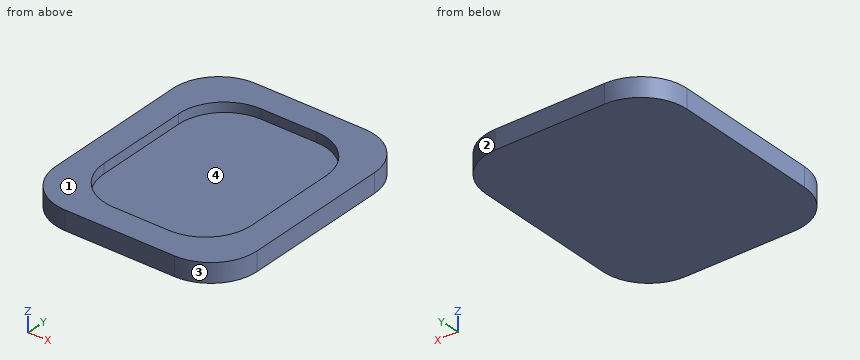
from build123d import *

# Parameters (mm, degrees)
F1_DEPTH = 5
F2_W     = 38.5
F2_H     = 48.5
F3_DEPTH = 2.5
F4_R     = 12


with BuildPart() as f1:
    # F0 (on Top) → F1 (new body)
    with BuildSketch(Plane.XY):
        with BuildLine():
            Line((40.5, 0), (12, 0))
            ThreePointArc((12, 0), (3.514719, -3.514719), (0, -12))
            Line((0, -12), (0, -50.5))
            ThreePointArc((0, -50.5), (3.514719, -58.985281), (12, -62.5))
            Line((12, -62.5), (40.5, -62.5))
            ThreePointArc((40.5, -62.5), (48.985281, -58.985281), (52.5, -50.5))
            Line((52.5, -50.5), (52.5, -12))
            ThreePointArc((52.5, -12), (48.985281, -3.514719), (40.5, 0))
        make_face()
    extrude(amount=F1_DEPTH)

    # F2 (on face) → F3 (cut)
    with BuildSketch(Plane.XY.offset(5)):
        with Locations((26.25, -31.25)):
            Rectangle(F2_W, F2_H)
    extrude(amount=-F3_DEPTH, mode=Mode.SUBTRACT)

    # F4
    f4_edges = [f1.edges().sort_by_distance(p)[0] for p in [
        (7, -7, 3.75),
        (45.5, -7, 3.75),
        (7, -55.5, 3.75),
        (45.5, -55.5, 3.75),
    ]]
    fillet(f4_edges, radius=F4_R)


solid = f1.part
Geometry check sheet. Reference: the model listing, model coordinates, mm. Face numbers are marked on the shaded views. Round coordinates to 2 decimals unless told otherwise and drop trailing zeros. Order: outer loops, then holes, each group sorted by start corner. A loop starts at its lowest first (then second) coordinate and runs counter-clockwise, first axis right, second up. Notation, with made-up numbers: M 23,19.25 L 65,19.25 A33 ccw 65,51.25 Z; hole C -14.5,16.25 d2. An arc over 180 degrees is marked long. Write each question's results on one line, items separated by ' | '. Start each with the question number.
1. Cross-section at B-B on x = 32.5. Record the boundary of the cut face in (y, z).
2. Cross-section at D-D on x = 48. Record the boundary of the cut face in (y, z), plus the area to 3 significant figures.
3. Cross-section at A-A on z = 3.3. Record the boundary of the cut face in (x, y), plus the area to 3 significant figures.
4. Go/stop test with flat-tipped pins: P1, Ø1, axis at x = 20, z = 4, coming from the +Y side; P2, Ø1.5, axis at x = 10.5, y = -28, coming from the +Z side. Record where each tip stops, or that it passes through.
5. Material ranges on L1, parallel to Y at x = 28.5, z = 4.5; L2, parallel to X at y = -33.5, z = 3; L3, parallel to Z at x = 9, y = -32, recorded low to high. Write a range as from..to.
6. Draft check along Y on the marked faces 1, 2, 3 and 4. Enter one of: pulls with the +Y half, pulls with the -Y half, needs draft (parallel to the pull), parting line crosses it, or undercut.
7. Cross-section at C-C on y = -25. Record the boundary of the cut face in (x, z).
Resolved:
1) outline: M -62.5,0 L 0,0 L 0,5 L -7,5 L -7,2.5 L -55.5,2.5 L -55.5,5 L -62.5,5 Z
2) outline: M -59.87,0 L -2.63,0 L -2.63,5 L -59.87,5 Z | area: 286 mm2
3) outline: M 0,-50.5 A12 ccw 12,-62.5 L 40.5,-62.5 A12 ccw 52.5,-50.5 L 52.5,-12 A12 ccw 40.5,0 L 12,0 A12 ccw 0,-12 Z; hole M 7,-43.5 A12 ccw 19,-55.5 L 33.5,-55.5 A12 ccw 45.5,-43.5 L 45.5,-19 A12 ccw 33.5,-7 L 19,-7 A12 ccw 7,-19 Z | area: 1,410 mm2
4) P1: y = 0 | P2: z = 2.5
5) L1: -62.5..-55.5, -7..0 | L2: 0..7, 45.5..52.5 | L3: 0..2.5
6) face 1: needs draft | face 2: pulls with the +Y half | face 3: pulls with the -Y half | face 4: undercut
7) outline: M 0,0 L 52.5,0 L 52.5,5 L 45.5,5 L 45.5,2.5 L 7,2.5 L 7,5 L 0,5 Z
